from build123d import *

# Parameters (mm, degrees)
SKETCH1_W                   = 45
SKETCH1_H                   = 14.46
BOSS_EXTRUDE1_DEPTH         = 3
F_1_4_0_25_DIAMETER_HOLE1_D = 6.35
SKETCH5_W                   = 24.2
SKETCH5_H                   = 37.04
BOSS_EXTRUDE2_DEPTH         = 3
SKETCH6_W                   = 10
SKETCH6_H                   = 30
BOSS_EXTRUDE3_DEPTH         = 5
BOSS_EXTRUDE4_START         = -29.2
SKETCH7_W                   = 10
SKETCH7_H                   = 30
BOSS_EXTRUDE4_DEPTH         = 5
SKETCH12_W                  = 24.2
SKETCH12_H                  = 20.5
CUT_EXTRUDE1_DEPTH          = 3
M5_CLEARANCE_HOLE1_D        = 5.5
FILLET3_R                   = 2.5
FILLET4_R                   = 2.5


with BuildPart() as part:
    # Sketch1 → Boss-Extrude1 (new body)
    with BuildSketch(Plane.XY):
        with Locations((13.988651535, -1.802042724)):
            Rectangle(SKETCH1_W, SKETCH1_H)
    extrude(amount=BOSS_EXTRUDE1_DEPTH)

    # 1/4 (0.25) Diameter Hole1 (through all)
    with Locations(Plane(origin=(0, 0, 0), x_dir=(-1, 0, 0), z_dir=(0, 0, -1))):
        with Locations((-26.488651535, -1.532042724), (-1.488651535, -1.532042724)):
            Hole(F_1_4_0_25_DIAMETER_HOLE1_D / 2)

    # Sketch5 → Boss-Extrude2 (add)
    with BuildSketch(Plane(origin=(0, 0, 0), x_dir=(-1, 0, 0), z_dir=(0, 0, -1))):
        with Locations((-13.988651535, 23.947957276)):
            Rectangle(SKETCH5_W, SKETCH5_H)
    extrude(amount=-BOSS_EXTRUDE2_DEPTH)

    # Sketch6 → Boss-Extrude3 (add)
    with BuildSketch(Plane.ZY.offset(-1.888651535)):
        with Locations((-2, 27.467957276)):
            Rectangle(SKETCH6_W, SKETCH6_H)
    extrude(amount=BOSS_EXTRUDE3_DEPTH)

    # Sketch7 → Boss-Extrude4 (add)
    with BuildSketch(Plane.ZY.offset(3.111348465).offset(BOSS_EXTRUDE4_START)):
        with Locations((-2, 27.467957276)):
            Rectangle(SKETCH7_W, SKETCH7_H)
    extrude(amount=-BOSS_EXTRUDE4_DEPTH)

    # Sketch12 → Cut-Extrude1 (cut)
    with BuildSketch(Plane(origin=(0, 0, 0), x_dir=(-1, 0, 0), z_dir=(0, 0, -1))):
        with Locations((-13.988651535, 32.217957276)):
            Rectangle(SKETCH12_W, SKETCH12_H)
    extrude(amount=-CUT_EXTRUDE1_DEPTH, mode=Mode.SUBTRACT)

    # M5 Clearance Hole1 (through all)
    with Locations(Plane.ZY.offset(3.111348465)):
        with Locations((-0.5, 37.467957276), (-0.5, 27.467957276)):
            Hole(M5_CLEARANCE_HOLE1_D / 2)

    # Fillet3
    fillet3_edges = [part.edges().sort_by_distance(p)[0] for p in [
        (-8.511348465, 5.427957276, 1.5),
        (36.488651535, 5.427957276, 1.5),
        (36.488651535, -9.032042724, 1.5),
        (-8.511348465, -9.032042724, 1.5),
    ]]
    fillet(fillet3_edges, radius=FILLET3_R)

    # Fillet4
    fillet4_edges = [part.edges().sort_by_distance(p)[0] for p in [
        (1.888651535, 5.427957276, 1.5),
        (26.088651535, 5.427957276, 1.5),
        (26.088651535, 12.467957276, 1.5),
        (1.888651535, 12.467957276, 1.5),
        (31.088651535, 12.467957276, -2),
        (-3.111348465, 12.467957276, -2),
        (28.588651535, 12.467957276, -7),
        (-0.611348465, 12.467957276, -7),
    ]]
    fillet(fillet4_edges, radius=FILLET4_R - 0.0001)  # a hair under: the kernel refuses the full size


solid = part.part
Build history of the part. All positions in model axes, mm. A direction names the side the tool comes from. Coordinates: 2 decimals unless noted, no trailing zeros. Write each loop counter-clockwise with the first axis right and the second up, starting at its lowest first coordinate (ties: lowest second). Pieces come first, ordered by that corner, then holes.
(1) Cut at D-D on y = 26.5. List the corners of the cut face in (x, z), and give its area (3 significant figures).
(2) Cut at B-B on y = 20. List the corners of the cut face in (x, z), and give its area (3 significant figures).
(3) 3-axis set-ups, long thin cutter, end or side, ignore diameter. For faces 4 (the flat face through (-3.111, 29, -3)), 5 (the cylindrical face through (-2.4, 13.22, -1.93)), 6 (the cylindrical face through (27, 6, 2)), 7 (the flat face through (1, 12.468, -2)): which of +Z, -Z, +X, -X, +Y, -Y reach the whole face in a straight line?
(4) Cut at C-C on x = 4. List the corners of the cut face in (y, z), and give its area (3 significant figures).
(5) Drill centre lines: line 1 (Y direction, x = -0.1, z = -0.5); line 2 (X direction, y = 33, z = -0.25); line 3 (Y direction, x = -0.5, z = 2). Where is each one in solid material? Low to high.
(6) Pin check, flat tips, straight feed: pin 1 Ø1.3 at (x, z) = (27, -2) entering from -Y; pin 2 Ø1.5 at (y, z) = (0, -1.5) entering from +X; pin 3 Ø3 at (y, z) = (22.5, 0.5) entering from -X; pin 4 Ø4 at (y, z) = (32.5, -2.5) entering from +X. Stop position of each tip, or through.
(7) Mould opens along Y. For faces 1 (the cylindrical face through (1.176, 11.716, 1.521)), 2 (the flat face through (14, 11, 3)), 3 (the cylindrical face through (-0.09, 13.18, -6.25)) say: pulls with the +Y half, pulls with the -Y half, needs draft (parallel to the pull), parting line crosses it, or undercut.
(8) Cut at A-A on x = 28. List the corners of the cut face in (y, z), and give its area (3 significant figures).
Working result:
1. outline: (-3.11, -7) - (1.89, -7) - (1.89, -3.07) - (-3.11, -3.07) - close; (-3.11, 2.07) - (1.89, 2.07) - (1.89, 3) - (-3.11, 3) - close; (26.09, -7) - (31.09, -7) - (31.09, -3.07) - (26.09, -3.07) - close; (26.09, 2.07) - (31.09, 2.07) - (31.09, 3) - (26.09, 3) - close
1. area: 48.5 mm2
2. outline: (-3.11, -7) - (1.89, -7) - (1.89, 0) - (26.09, 0) - (26.09, -7) - (31.09, -7) - (31.09, 3) - (-3.11, 3) - close
2. area: 173 mm2
3. face 4: +Z, -Z, -X, +Y
3. face 5: +Z, -Z, -X
3. face 6: +Z, -Z, +X
3. face 7: -Z, +X, -X, -Y
4. outline: (-9.03, 0) - (-3.47, 0) - (-3.47, 3) - (-9.03, 3) - close; (0.41, 0) - (21.97, 0) - (21.97, 3) - (0.41, 3) - close
4. area: 81.3 mm2
5. line 1: y = 12.47 to 24.72, 30.22 to 34.72, 40.22 to 42.47
5. line 2: x = -3.11 to 1.89, 26.09 to 31.09
5. line 3: y = -9.03 to -4.01, 0.94 to 5.43, 12.47 to 26.32, 28.61 to 36.32, 38.61 to 42.47
6. pin 1: stops at y = 12.47
6. pin 2: passes through
6. pin 3: stops at x = -3.11
6. pin 4: stops at x = 31.09
7. face 1: undercut
7. face 2: needs draft
7. face 3: pulls with the -Y half
8. outline: (-9.03, 0) - (-4.32, 0) - (-4.32, 3) - (-9.03, 3) - close; (1.26, 0) - (5.5, 0) - (5.5, 3) - (1.26, 3) - close; (12.4, 0) - (12.47, 0) - (12.47, -4.5) arc R2.5 ccw to (14.97, -7) - (42.47, -7) - (42.47, 3) - (12.4, 3) - close; hole circle Ø5.5 at (27.47, -0.5); hole circle Ø5.5 at (37.47, -0.5)
8. area: 278 mm2
